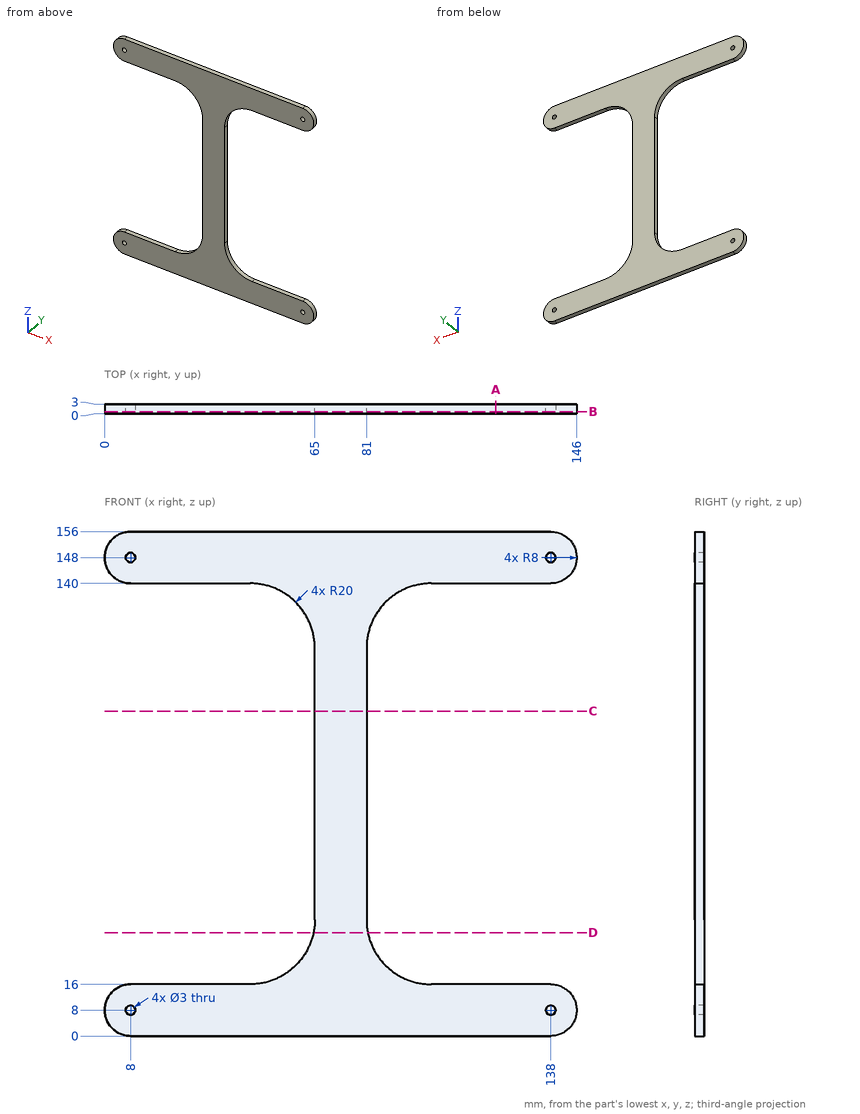
Geometry: see drawing. Coordinates: mm, zero at the bounding-box minimum. Give positions to 0.01 mm unless a question says otherwise; leave off trailing zeros. Order: outer loops, then holes, each group sorted by start corner. A loop starts at its lowest first (then second) coordinate and runs counter-clockwise, first axis right, second up.
Q1. Section C-C on z = 100.5. Output: boundary loops of the cut face in (x, y).
Checked values:
outline: (65, 0) - (81, 0) - (81, 3) - (65, 3) - close
Q2. Contact query for a flat-ended pin moving along its axis: pin 1 Ø0.9 at (y, z) = (2, 75.5) entering from +X. Output: stop coordinate, or through.
Checked values:
pin 1: stops at x = 81
Q3. Section A-A on x = 121. Output: boundary loops of the cut face in (y, z).
Checked values:
outline: (0, 0) - (3, 0) - (3, 16) - (0, 16) - close; (0, 140) - (3, 140) - (3, 156) - (0, 156) - close
Q4. Section B-B on y = 0.65. Output: boundary loops of the cut face in (x, z), and give its area (3 significant figures).
Checked values:
outline: (8, 0) - (138, 0) arc R8 ccw to (138, 16) - (101, 16) arc R20 cw to (81, 36) - (81, 120) arc R20 cw to (101, 140) - (138, 140) arc R8 ccw to (138, 156) - (8, 156) arc R8 ccw to (8, 140) - (45, 140) arc R20 cw to (65, 120) - (65, 36) arc R20 cw to (45, 16) - (8, 16) arc R8 ccw to start; hole circle Ø3 at (8, 8); hole circle Ø3 at (8, 148); hole circle Ø3 at (138, 8); hole circle Ø3 at (138, 148)
area: 6,860 mm2
Q5. Ray query, probe 1 along X at (y, z) = (0.6, 8); probe 2 along Z at (x, y) = (8, 0.8); probe 3 along X at (y, z) = (2.5, 42). Return the intervals inside material, ascending.
Checked values:
probe 1: x = 0 to 6.5, 9.5 to 136.5, 139.5 to 146
probe 2: z = 0 to 6.5, 9.5 to 16, 140 to 146.5, 149.5 to 156
probe 3: x = 65 to 81
Q6. Section D-D on z = 32. Output: boundary loops of the cut face in (x, y), and give its area (3 significant figures).
Checked values:
outline: (64.6, 0) - (81.4, 0) - (81.4, 3) - (64.6, 3) - close
area: 50.4 mm2
